Can you work these out from the model? Positions are in its coordinate system, mm. Face numbers are marked on the shaded views. A direction names the side the tool comes from. Round coordinates to 2 decimals unless told otherwise and drop trailing zeros. Loops run counter-clockwise (first coordinate to the right, second up) from the corner with the lowest first, then second, coordinate; pieces in that order, holes last.
```python
from build123d import *

# Parameters (mm, degrees)
MAIN_PROFILE_SKETCH_R     = 8.5
MAIN_EXTRUSION_DEPTH      = 2
DETAIL_EXTRUSION_2_DEPTH  = 31.5
DETAIL_EXTRUSION_3_DEPTH  = 0.5
DETAIL_PROFILE_4_SKETCH_R = 6
DETAIL_EXTRUSION_4_DEPTH  = 8


with BuildPart() as part:
    # Main Profile Sketch → Main Extrusion (new body)
    with BuildSketch(Plane(origin=(0, -123, 0), x_dir=(-1, 0, 0), z_dir=(0, -1, 0))):
        with Locations(Location((56.291651246, 0, 0), (0, 0, 90))):
            Circle(MAIN_PROFILE_SKETCH_R)
    extrude(amount=MAIN_EXTRUSION_DEPTH)

    # Detail Profile 2 Sketch → Detail Extrusion 2 (add)
    with BuildSketch(Plane(origin=(0, -125, 0), x_dir=(-1, 0, 0), z_dir=(0, -1, 0))):
        with BuildLine():
            ThreePointArc((51.384442087, -3.452433674), (62.011933361, 1.81062766), (50.291651246, 0))
            ThreePointArc((50.291651246, 0), (50.571369131, -1.81062766), (51.384442087, -3.452433674))
        make_face()
    extrude(amount=DETAIL_EXTRUSION_2_DEPTH)

    # Detail Profile 3 Sketch → Detail Extrusion 3 (add)
    with BuildSketch(Plane(origin=(0, -156.5, 0), x_dir=(-1, 0, 0), z_dir=(0, -1, 0))):
        with BuildLine():
            ThreePointArc((51.384442087, -3.452433674), (62.011933361, 1.81062766), (50.291651246, 0))
            ThreePointArc((50.291651246, 0), (50.571369131, -1.81062766), (51.384442087, -3.452433674))
        make_face()
    extrude(amount=DETAIL_EXTRUSION_3_DEPTH)

    # Detail Profile 4 Sketch → Detail Extrusion 4 (add)
    with BuildSketch(Plane(origin=(0, -157, 0), x_dir=(-1, 0, 0), z_dir=(0, -1, 0))):
        with Locations(Location((56.291651246, 0, 0), (0, 0, 90))):
            Circle(DETAIL_PROFILE_4_SKETCH_R)
    extrude(amount=DETAIL_EXTRUSION_4_DEPTH)


solid = part.part
```
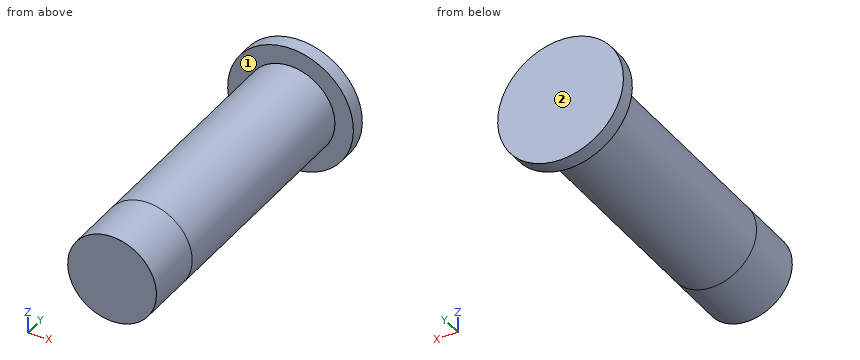
(1) Suppose I cut it at D-D (x = -54). Write out the boundary of the cut face in (y, z), then the cut area to 3 significant figures.
(2) Which directions (+Z, -Z, +X, -X, +Y, -Y) give clear straight access to the entire face, cutting with the end or side of a thin tool? Please do the marked faces 1 and 2.
(3) Suppose I cut it at B-B (x = -58.25). Write out the boundary of the cut face in (y, z), then the cut area to 3 significant figures.
(4) Suppose I cut it at A-A (z = 0). Write out the boundary of the cut face in (x, y), then the cut area to 3 significant figures.
(5) If I drill on line 1 (Y direction, x = -53, z = -7); line 2 (X direction, y = -137.5, z = -5.5); line 3 (X direction, y = -155.5, z = 1.25), over which ranges is the centre line in solid material (lowest first)?
(6) Suppose I cut it at C-C (y = -160). Write out the boundary of the cut face in (x, z), then the cut area to 3 significant figures.
(7) For pin 1 (3 mm diameter, centred on y = -152.5, z = 3, fed in from +X); pin 2 (4 mm diameter, centred on x = -60, y = -160.5, fed in from +Z); pin 3 (2 mm diameter, centred on x = -53.5, y = -144, fed in from +Z), each with a flat end and sliding along its axis, tell me the tip position at first contact or that it passes through.
Check result:
1. outline: (-165, -5.55) - (-125, -5.55) - (-125, -8.19) - (-123, -8.19) - (-123, 8.19) - (-125, 8.19) - (-125, 5.55) - (-165, 5.55) - close
1. area: 476 mm2
2. face 1: -Y
2. face 2: +Z, -Z, +X, -X, +Y
3. outline: (-165, -5.67) - (-125, -5.67) - (-125, -8.27) - (-123, -8.27) - (-123, 8.27) - (-125, 8.27) - (-125, 5.67) - (-165, 5.67) - close
3. area: 487 mm2
4. outline: (-64.79, -125) - (-62.29, -125) - (-62.29, -165) - (-50.29, -165) - (-50.29, -125) - (-47.79, -125) - (-47.79, -123) - (-64.79, -123) - close
4. area: 514 mm2
5. line 1: y = -125 to -123
5. line 2: x = -58.69 to -53.89
5. line 3: x = -62.16 to -50.42
6. outline: circle Ø12 at (-56.29, 0)
6. area: 113 mm2
7. pin 1: stops at x = -50.48
7. pin 2: stops at z = 5.75
7. pin 3: stops at z = 5.73
